Geometry check sheet. Reference: drawing and pictorial views, mm from the part's lowest x, y, z. A direction names the side the tool comes from. Round coordinates to 2 decimals unless told otherwise and drop trailing zeros. Order: outer loops, then holes, each group sorted by start corner. A loop starts at its lowest first (then second) coordinate and runs counter-clockwise, first axis right, second up.
(1) Sectioned sample at A-A (y = 8). Record the boundary of the cut face in (x, z).
(2) Set-up check for the marked faces 5, 6 and 7: record each of +Z, -Z, +X, -X, +Y, -Y from which the full face is reachable in a straight line by a thin tool's end or side.
(3) Sectioned sample at C-C (x = 17.5). Record the boundary of the cut face in (y, z).
(4) Go/stop test with flat-tipped pins: pin 1 (2.5 mm diameter, centred on x = 6, z = 3.5, fed in from -Y); pin 2 (3 mm diameter, centred on x = 27, z = 5, fed in from -Y). Record where each tip stops, or that it passes through.
(5) Release check for a two-part mould opening along X. For the marked faces 1, 2, 3 and 4 record: +X half, -X half, draft (parallel to the pull), parting line (faces both ways), or undercut.
(6) Material ranges on line 1 along Z through (x, y) = (32.5, 17.75); line 2 along X through (y, z) = (4.5, 4); line 3 along X through (y, z) = (8.25, 3.5), recorded low to high.
(7) Sectioned sample at D-D (y = 14). Record the boundary of the cut face in (x, z).
(8) Sectioned sample at B-B (z = 5). Give the number of separate pieces and of enclosed holes in the cut face, plus the area to 3 significant figures.
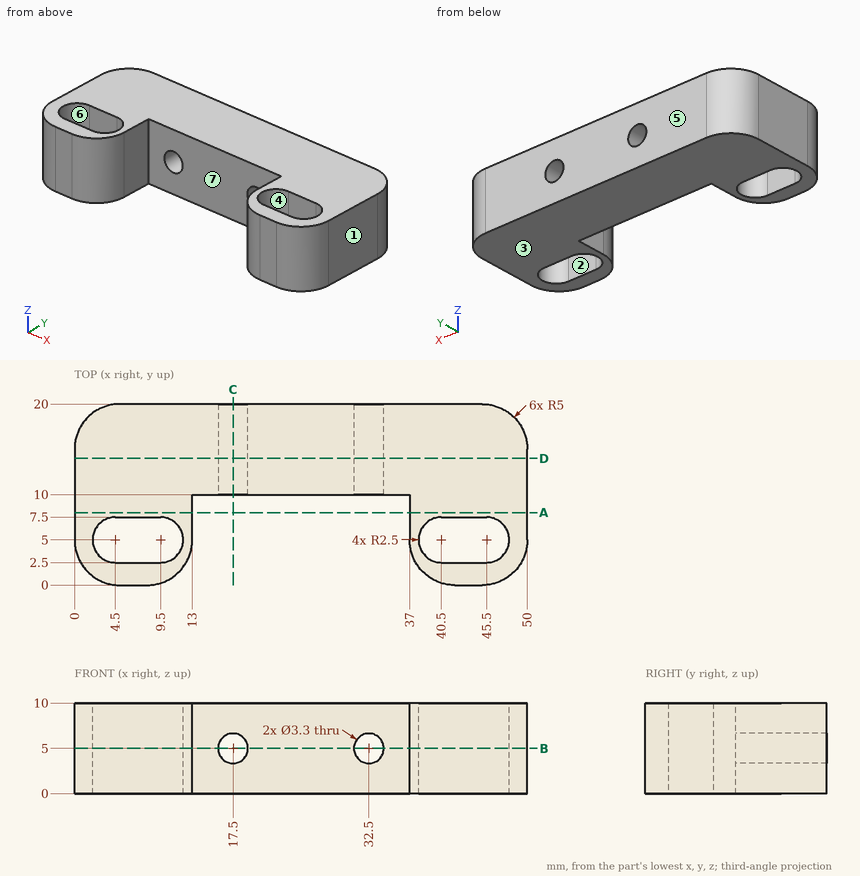
Answer below:
1. outline: (0, 0) - (13, 0) - (13, 10) - (0, 10) - close; (37, 0) - (50, 0) - (50, 10) - (37, 10) - close
2. face 5: +Z, -Z, +X, -X, +Y
2. face 6: +Z, -Z
2. face 7: +Z, -Z, -Y
3. outline: (10, 0) - (20, 0) - (20, 3.35) - (10, 3.35) - close; (10, 6.65) - (20, 6.65) - (20, 10) - (10, 10) - close
4. pin 1: stops at y = 0
4. pin 2: stops at y = 10
5. face 1: +X half
5. face 2: undercut
5. face 3: draft
5. face 4: undercut
6. line 1: z = 0 to 3.35, 6.65 to 10
6. line 2: x = 0.03 to 2.05, 11.95 to 12.97, 37.03 to 38.05, 47.95 to 49.97
6. line 3: x = 0 to 13, 37 to 50
7. outline: (0, 0) - (50, 0) - (50, 10) - (0, 10) - close; hole circle Ø3.3 at (17.5, 5); hole circle Ø3.3 at (32.5, 5)
8. separate pieces: 3
8. enclosed holes: 2
8. area: 573 mm2
